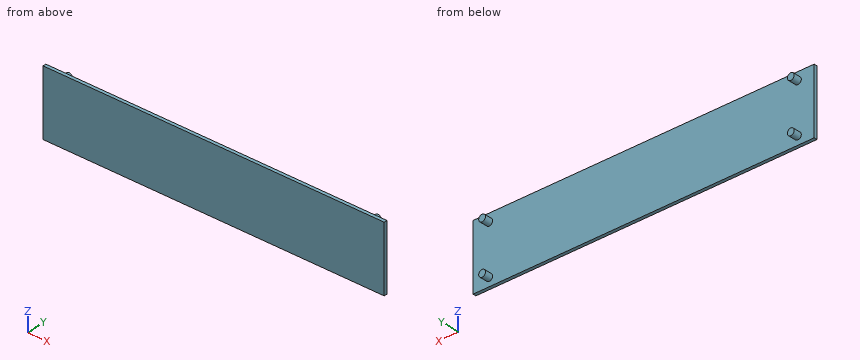
from build123d import *

# Parameters (mm, degrees)
SKETCH_1_W      = 210
SKETCH_1_H      = 40
EXTRUDE_1_DEPTH = 2
SKETCH_2_R      = 2.1
EXTRUDE_2_DEPTH = 5


with BuildPart() as part:
    # 草图1 → 凸台-拉伸1 (new body)
    with BuildSketch(Plane(origin=(0, 0, 0), x_dir=(1, 0, 0), z_dir=(0, 1, 0))):
        Rectangle(SKETCH_1_W, SKETCH_1_H)
    extrude(amount=EXTRUDE_1_DEPTH)

    # 草图2 → 凸台-拉伸2 (add)
    with BuildSketch(Plane(origin=(0, 2, 0), x_dir=(1, 0, 0), z_dir=(0, 1, 0))):
        with Locations(Location((95, -15, 0), (0, 0, 270))):
            Circle(SKETCH_2_R)
        with Locations(Location((95, 15, 0), (0, 0, 270))):
            Circle(SKETCH_2_R)
        with Locations(Location((-95, 15, 0), (0, 0, 270))):
            Circle(SKETCH_2_R)
        with Locations(Location((-95, -15, 0), (0, 0, 270))):
            Circle(SKETCH_2_R)
    extrude(amount=EXTRUDE_2_DEPTH)


solid = part.part
Could you check a few things on this model? Use its own coordinates, in mm. Give positions to 0.01 mm unless a question says otherwise; leave off trailing zeros. Write each loop counter-clockwise with the first axis right and the second up, starting at its lowest first coordinate (ties: lowest second). Pieces come first, ordered by that corner, then holes. Notation, with made-up numbers: (68, 79) - (76, 79) arc R30 ccw to (76, 106) - close; hole circle Ø9 at (43.5, 29.25). An arc over 180 degrees is marked (long way). Use CSV: the item, a comma, the result in double quotes. Start each with the question number.
Item 1: I want a section at B-B, the plane y = 4.5. Please give me the cut outline in (x, z).
Item 2: I want a section at C-C, the plane z = 15. Please give me the cut outline in (x, y), then the cut area to 3 significant figures.
Item 3: I want a section at D-D, the plane z = -9. Please give me the cut outline in (x, y).
Item 4: I want a section at A-A, the plane x = -95. Please give me the cut outline in (y, z), then the cut area to 3 significant figures.
Item 5: I'm going to push flat-ended pins straight in: pin 1 (4 mm diameter, centred on y = 3, z = 8, fed in from -X); pin 2 (5 mm diameter, centred on x = -33.5, z = 7, fed in from +Y). Where does each tip first touch, or does it pass through?
Item 6: If I drill on line 1 along Y through (x, z) = (66, -10); line 2 along X through (y, z) = (2.5, -14), over which ranges is the centre line in solid material (lowest first)?
Findings:
1,outline,"circle Ø4.2 at (-95, -15); circle Ø4.2 at (-95, 15); circle Ø4.2 at (95, -15); circle Ø4.2 at (95, 15)"
2,outline,"(-105, 0) - (105, 0) - (105, 2) - (97.1, 2) - (97.1, 7) - (92.9, 7) - (92.9, 2) - (-92.9, 2) - (-92.9, 7) - (-97.1, 7) - (-97.1, 2) - (-105, 2) - close"
2,area,"462 mm2"
3,outline,"(-105, 0) - (105, 0) - (105, 2) - (-105, 2) - close"
4,outline,"(0, -20) - (2, -20) - (2, -17.1) - (7, -17.1) - (7, -12.9) - (2, -12.9) - (2, 12.9) - (7, 12.9) - (7, 17.1) - (2, 17.1) - (2, 20) - (0, 20) - close"
4,area,"122 mm2"
5,pin 1,"stops at x = -105"
5,pin 2,"stops at y = 2"
6,line 1,"y = 0 to 2"
6,line 2,"x = -96.85 to -93.15, 93.15 to 96.85"
